The model under review builds one solid part; all positions refer to its coordinate system, in mm. Face numbers are marked on the shaded views. Round coordinates to 2 decimals unless told otherwise and drop trailing zeros. Order: outer loops, then holes, each group sorted by start corner. A loop starts at its lowest first (then second) coordinate and runs counter-clockwise, first axis right, second up.
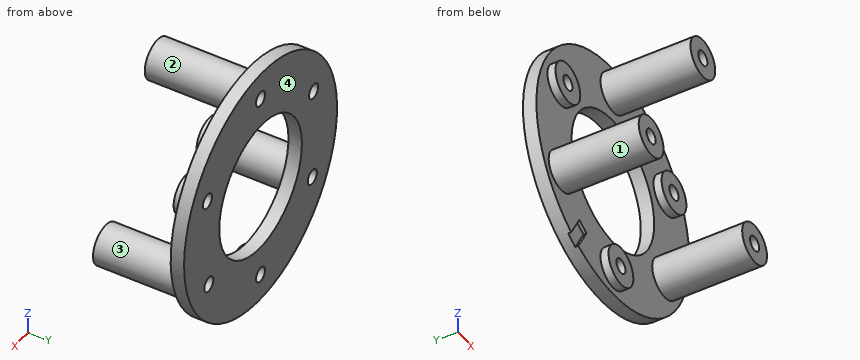
from build123d import *

# Parameters (mm, degrees)
SKETCH_1_R          = 18.5
SKETCH_1_R_2        = 10
SKETCH_1_R_3        = 1.1
EXTRUDE_1_DEPTH     = 2
EXTRUDE_START       = -3.2
SKETCH_2_R          = 3
SKETCH_2_R_2        = 1.1
EXTRUDE_2_DEPTH     = 1.2
SKETCH_3_R          = 1.1
CUT_EXTRUDE_1_DEPTH = 27.357921011
SKETCH_4_R          = 3
SKETCH_4_R_2        = 1.1
EXTRUDE_3_DEPTH     = 13.4
CUT_EXTRUDE_2_DEPTH = 0.44


with BuildPart() as part:
    # Эскиз1 → Бобышка-Вытянуть1 (new body)
    with BuildSketch(Plane(origin=(0, 0, 0), x_dir=(1, 0, 0), z_dir=(0, 1, 0))):
        with Locations(Location((0, 0, 0), (0, 0, 270))):
            Circle(SKETCH_1_R)
        with Locations(Location((0, 0, 0), (0, 0, 270))):
            Circle(SKETCH_1_R_2, mode=Mode.SUBTRACT)
        with Locations(Location((0, 14.46, 0), (0, 0, 270))):
            Circle(SKETCH_1_R_3, mode=Mode.SUBTRACT)
        with Locations(Location((12.837810469, -6.654488888, 0), (0, 0, 270))):
            Circle(SKETCH_1_R_3, mode=Mode.SUBTRACT)
        with Locations(Location((-12.837810469, -6.654488888, 0), (0, 0, 270))):
            Circle(SKETCH_1_R_3, mode=Mode.SUBTRACT)
    extrude(amount=EXTRUDE_1_DEPTH)

    # Эскиз2 → Бобышка-Вытянуть2 (add)
    # profile 1 of 3: a face of its own
    with BuildSketch(Plane(origin=(0, 2, 0), x_dir=(1, 0, 0), z_dir=(0, 1, 0)).offset(EXTRUDE_START)):
        with Locations(Location((0, 14.46, 0), (0, 0, 270))):
            Circle(SKETCH_2_R)
        with Locations(Location((0, 14.46, 0), (0, 0, 270))):
            Circle(SKETCH_2_R_2, mode=Mode.SUBTRACT)
    # profile 2 of 3: a face of its own
    with BuildSketch(Plane(origin=(0, 2, 0), x_dir=(1, 0, 0), z_dir=(0, 1, 0)).offset(EXTRUDE_START)):
        with Locations(Location((-12.837810469, -6.654488888, 0), (0, 0, 270))):
            Circle(SKETCH_2_R)
        with Locations(Location((-12.837810469, -6.654488888, 0), (0, 0, 270))):
            Circle(SKETCH_2_R_2, mode=Mode.SUBTRACT)
    # profile 3 of 3: a face of its own
    with BuildSketch(Plane(origin=(0, 2, 0), x_dir=(1, 0, 0), z_dir=(0, 1, 0)).offset(EXTRUDE_START)):
        with Locations(Location((12.837810469, -6.654488888, 0), (0, 0, 270))):
            Circle(SKETCH_2_R)
        with Locations(Location((12.837810469, -6.654488888, 0), (0, 0, 270))):
            Circle(SKETCH_2_R_2, mode=Mode.SUBTRACT)
    extrude(amount=EXTRUDE_2_DEPTH)

    # Эскиз3 → Вырез-Вытянуть1 (cut, through all)
    with BuildSketch(Plane(origin=(0, 2, 0), x_dir=(1, 0, 0), z_dir=(0, 1, 0))):
        with Locations(Location((-12.522727339, 7.23, 0), (0, 0, 270))):
            Circle(SKETCH_3_R)
        with Locations(Location((12.522727339, 7.23, 0), (0, 0, 270))):
            Circle(SKETCH_3_R)
        with Locations(Location((0, -14.46, 0), (0, 0, 270))):
            Circle(SKETCH_3_R)
    extrude(amount=-CUT_EXTRUDE_1_DEPTH, mode=Mode.SUBTRACT)

    # Эскиз4 → Бобышка-Вытянуть3 (add)
    # profile 1 of 3: a face of its own
    with BuildSketch(Plane.XZ):
        with Locations(Location((-12.522727339, -7.23, 0), (0, 0, 90))):
            Circle(SKETCH_4_R)
        with Locations(Location((-12.522727339, -7.23, 0), (0, 0, 90))):
            Circle(SKETCH_4_R_2, mode=Mode.SUBTRACT)
    # profile 2 of 3: a face of its own
    with BuildSketch(Plane.XZ):
        with Locations(Location((0, 14.46, 0), (0, 0, 90))):
            Circle(SKETCH_4_R)
        with Locations(Location((0, 14.46, 0), (0, 0, 90))):
            Circle(SKETCH_4_R_2, mode=Mode.SUBTRACT)
    # profile 3 of 3: a face of its own
    with BuildSketch(Plane.XZ):
        with Locations(Location((12.522727339, -7.23, 0), (0, 0, 90))):
            Circle(SKETCH_4_R)
        with Locations(Location((12.522727339, -7.23, 0), (0, 0, 90))):
            Circle(SKETCH_4_R_2, mode=Mode.SUBTRACT)
    extrude(amount=EXTRUDE_3_DEPTH)

    # Эскиз5 → Вырез-Вытянуть2 (cut)
    with BuildSketch(Plane.XZ):
        Polygon((-8.383974596, -16.52146997), (-6.383974596, -13.057368355), (-8.116025404, -12.057368355), (-10.116025404, -15.52146997), align=None)
    extrude(amount=-CUT_EXTRUDE_2_DEPTH, mode=Mode.SUBTRACT)


solid = part.part
(1) We need section B-B (y = -11.5). Give the boundary of the cut face in (x, z), and give its area (3 significant figures).
(2) We need section A-A (z = 0). Give the boundary of the cut face in (x, y).
(3) To check wall thickness, follow L1, parallel to X at y = -4.25, z = -7.23; L2, parallel to Y at x = -13.5, z = 4; L3, parallel to X at y = 1.45, z = 14.46. State the ranges of each line that lie inside material, in increasing order.
(4) Clearance check with flat-ended pins moving along their axes: P1, Ø2.5, axis at x = 0, z = -14.46, coming from the +Y side; P2, Ø5, axis at x = 13, z = 6, coming from the -Y side; P3, Ø1, axis at x = 6.5, z = -5.5, coming from the -Y side; P4, Ø1.5, axis at y = -5.5, z = 12, coming from the -X side. State where each tip first meets the part, or that it passes through.
(5) We need section C-C (x = 5). Give the boundary of the cut face in (y, z), and give its area (3 significant figures).
(6) We need section D-D (z = -7.23). Give the boundary of the cut face in (x, y), and give its area (3 significant figures).
(7) The part is to be moulded in two halves that separate along X. For the marked faces 1, 2, 3 and 4, say which applies: pulls with the +X half, pulls with the -X half, needs draft (parallel to the pull), parting line crosses it, or undercut.
Verdict:
1. outline: circle Ø6 at (-12.52, -7.23); circle Ø6 at (0, 14.46); circle Ø6 at (12.52, -7.23); hole circle Ø2.2 at (-12.52, -7.23); hole circle Ø2.2 at (0, 14.46); hole circle Ø2.2 at (12.52, -7.23)
1. area: 73.4 mm2
2. outline: (-18.5, 0) - (-10, 0) - (-10, 2) - (-18.5, 2) - close; (10, 0) - (18.5, 0) - (18.5, 2) - (10, 2) - close
3. L1: x = -15.52 to -13.62, -11.42 to -9.52, 9.52 to 11.42, 13.62 to 15.52
3. L2: y = -1.2 to 2
3. L3: x = -11.54 to -1.1, 1.1 to 11.54
4. P1: stops at y = 2
4. P2: stops at y = -1.2
4. P3: passes through
4. P4: stops at x = -2.46
5. outline: (0, -17.81) - (2, -17.81) - (2, -8.66) - (0, -8.66) - close; (0, 8.66) - (2, 8.66) - (2, 17.81) - (0, 17.81) - close
5. area: 36.6 mm2
6. outline: (-17.03, 0) - (-15.52, 0) - (-15.52, -13.4) - (-13.62, -13.4) - (-13.62, 2) - (-17.03, 2) - close; (-11.42, -13.4) - (-9.52, -13.4) - (-9.52, 0) - (-6.91, 0) - (-6.91, 2) - (-11.42, 2) - close; (6.91, 0) - (9.52, 0) - (9.52, -13.4) - (11.42, -13.4) - (11.42, 2) - (6.91, 2) - close; (13.62, -13.4) - (15.52, -13.4) - (15.52, 0) - (17.03, 0) - (17.03, 2) - (13.62, 2) - close
6. area: 134 mm2
7. face 1: undercut
7. face 2: parting line crosses it
7. face 3: undercut
7. face 4: needs draft
